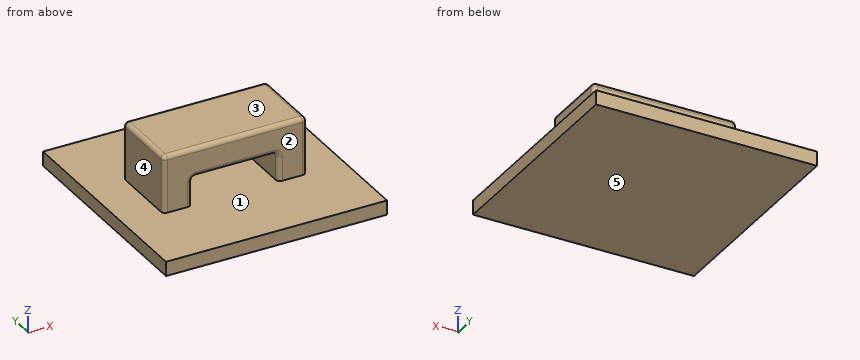
from build123d import *

# Parameters (mm, degrees)
F1_DEPTH = 3.175
F2_R     = 0.381
F3_W     = 19.558
F3_H     = 19.558
F4_DEPTH = 1.27


with BuildPart() as f1:
    # F0 (on Front) → F1 (new body, symmetric)
    with BuildSketch(Plane.XZ):
        Polygon((-3.81, -1.27), (-3.81, 1.27), (3.81, 1.27), (3.81, -1.27), (6.35, -1.27), (6.35, 3.81), (-6.35, 3.81), (-6.35, -1.27), align=None)
    extrude(amount=F1_DEPTH, both=True)

    # F2
    f2_edges = [f1.edges().sort_by_distance(p)[0] for p in [
        (0, 3.175, 3.81),
        (6.35, 0, 3.81),
        (0, -3.175, 3.81),
        (-6.35, 0, 3.81),
        (-6.35, -3.175, 1.27),
        (-6.35, 3.175, 1.27),
        (0, 3.175, 1.27),
        (-3.81, 3.175, 0),
        (3.81, 3.175, 0),
        (6.35, 3.175, 1.27),
        (6.35, -3.175, 1.27),
        (0, -3.175, 1.27),
        (-3.81, -3.175, 0),
        (3.81, -3.175, 0),
        (-3.81, 0, 1.27),
        (3.81, 0, 1.27),
    ]]
    fillet(f2_edges, radius=F2_R)

    # F3 (on face) → F4 (join)
    with BuildSketch(Plane(origin=(0, 0, -1.27), x_dir=(1, 0, 0), z_dir=(0, 0, -1))):
        Rectangle(F3_W, F3_H)
        with BuildLine():
            Line((3.81, -2.794), (3.81, 2.794))
            ThreePointArc((3.81, 2.794), (3.921592, 3.063408), (4.191, 3.175))
            Line((4.191, 3.175), (5.969, 3.175))
            ThreePointArc((5.969, 3.175), (6.238408, 3.063408), (6.35, 2.794))
            Line((6.35, 2.794), (6.35, -2.794))
            ThreePointArc((6.35, -2.794), (6.238408, -3.063408), (5.969, -3.175))
            Line((5.969, -3.175), (4.191, -3.175))
            ThreePointArc((4.191, -3.175), (3.921592, -3.063408), (3.81, -2.794))
        make_face(mode=Mode.SUBTRACT)
        with BuildLine():
            ThreePointArc((4.191, 3.175), (3.921592, 3.063408), (3.81, 2.794))
            Line((3.81, 2.794), (3.81, -2.794))
            ThreePointArc((3.81, -2.794), (3.921592, -3.063408), (4.191, -3.175))
            Line((4.191, -3.175), (5.969, -3.175))
            ThreePointArc((5.969, -3.175), (6.238408, -3.063408), (6.35, -2.794))
            Line((6.35, -2.794), (6.35, 2.794))
            ThreePointArc((6.35, 2.794), (6.238408, 3.063408), (5.969, 3.175))
            Line((5.969, 3.175), (4.191, 3.175))
        make_face()
    extrude(amount=F4_DEPTH)


solid = f1.part
Can you work these out from the model? Positions are in its coordinate system, mm. Face numbers are marked on the shaded views. A direction names the side the tool comes from. Give positions to 0.01 mm unless a question says otherwise; leave off trailing zeros. Order: outer loops, then holes, each group sorted by start corner. A loop starts at its lowest first (then second) coordinate and runs counter-clockwise, first axis right, second up. Notation, with made-up numbers: M -14.75,55.5 L 30.25,55.5 A22 cw 30.25,76.5 Z; hole C -15.5,40 d9. An arc over 180 degrees is marked long. One line per question, with ' | ' between items.
Item 1: We'd pull the mould along Z, two halves only. Please class the marked faces 1, 2 and 3: released by +Z, released by -Z, zero draft, split by the parting line, or undercut.
Answer block:
face 1: undercut | face 2: zero draft | face 3: released by +Z
Item 2: Please list where these lines run through material, in increasing order: L1, parallel to X at y = 0.5, z = 0.5; L2, parallel to Z at x = 3, y = -2; L3, parallel to Z at x = 9.25, y = -3.5.
Answer block:
L1: x = -6.35 to -3.81, 3.81 to 6.35 | L2: z = -2.54 to -1.27, 1.27 to 3.81 | L3: z = -2.54 to -1.27
Item 3: I'm going to push flat-ended pins straight in: pin 1 Ø4 at (x, y) = (-1, 4.5) entering from +Z; pin 2 Ø1.1 at (y, z) = (0, -0.5) entering from -X; pin 3 Ø1.1 at (y, z) = (-0.5, -0.5) entering from +X; pin 4 Ø2.5 at (x, z) = (1.5, 2) entering from -Y (3 decimals). Where does each tip first touch, or does it pass through?
Answer block:
pin 1: stops at z = 3.81 | pin 2: stops at x = -6.35 | pin 3: stops at x = 6.35 | pin 4: stops at y = -3.175
Item 4: For the marked faces 4 and 5, which set-ups out of +Z, -Z, +X, -X, +Y, -Y let a thin tool reach every point of the face, with its end or its side?
Answer block:
face 4: +Z, -X, +Y, -Y | face 5: -Z, +X, -X, +Y, -Y
Item 5: Suppose I cut it at A-A, the plane x = 0.75. Write out the boundary of the cut face in (y, z) (3 decimals).
Answer block:
outline: M -9.779,-2.54 L 9.779,-2.54 L 9.779,-1.27 L -9.779,-1.27 Z; M -3.175,1.651 A0.381 ccw -2.794,1.27 L 2.794,1.27 A0.381 ccw 3.175,1.651 L 3.175,3.429 A0.381 ccw 2.794,3.81 L -2.794,3.81 A0.381 ccw -3.175,3.429 Z
Item 6: Suppose I cut it at B-B, the plane z = -0.25. Write out the boundary of the cut face in (x, y) (3 decimals), then the cut area to 3 significant figures.
Answer block:
outline: M -6.35,-2.794 A0.381 ccw -5.969,-3.175 L -4.191,-3.175 A0.381 ccw -3.81,-2.794 L -3.81,2.794 A0.381 ccw -4.191,3.175 L -5.969,3.175 A0.381 ccw -6.35,2.794 Z; M 3.81,-2.794 A0.381 ccw 4.191,-3.175 L 5.969,-3.175 A0.381 ccw 6.35,-2.794 L 6.35,2.794 A0.381 ccw 5.969,3.175 L 4.191,3.175 A0.381 ccw 3.81,2.794 Z | area: 32.0 mm2
Item 7: Suppose I cut it at C-C, the plane y = -1. Write out the boundary of the cut face in (x, z).
Answer block:
outline: M -9.78,-2.54 L 9.78,-2.54 L 9.78,-1.27 L 6.35,-1.27 L 6.35,3.43 A0.38 ccw 5.97,3.81 L -5.97,3.81 A0.38 ccw -6.35,3.43 L -6.35,-1.27 L -9.78,-1.27 Z; hole M -3.81,-1.27 L 3.81,-1.27 L 3.81,0.89 A0.38 ccw 3.43,1.27 L -3.43,1.27 A0.38 ccw -3.81,0.89 Z
Item 8: Suppose I cut it at D-D, the plane y = 7.75. Write out the boundary of the cut face in (x, z), then the cut area to 3 significant figures.
Answer block:
outline: M -9.78,-2.54 L 9.78,-2.54 L 9.78,-1.27 L -9.78,-1.27 Z | area: 24.8 mm2
